Can you work these out from the model? Positions are in its coordinate system, mm. Give positions to 0.01 mm unless a question says otherwise; leave off trailing zeros. Loops run counter-clockwise (first coordinate to the right, second up) from the corner with the lowest first, then second, coordinate; pieces in that order, holes last. Notation, with made-up numbers: (56, -16.5) - (61, -16.5) arc R13 cw to (61, -8.5) - close; hole circle Ø8 at (15.5, 61.25). An arc over 180 degrees is marked (long way). Answer as a JSON object with one key per item and string values.
```python
from build123d import *

# Parameters (mm, degrees)
F0_R     = 6.35
F1_DEPTH = 2.54
F2_DEPTH = 25.4


with BuildPart() as f1:
    # F0 (on Top) → F1 (new body)
    with BuildSketch(Plane.XY):
        with BuildLine():
            ThreePointArc((1.98040625, 18.6275212343), (3.3011106094, 18.4393390607), (4.6050729167, 18.157639155))
            ThreePointArc((4.6050729167, 18.157639155), (6.310350892, 21.0006716461), (8.2563229167, 23.6846983968))
            ThreePointArc((8.2563229167, 23.6846983968), (6.9543084231, 24.0991576742), (5.63165625, 24.4421000352))
            ThreePointArc((5.63165625, 24.4421000352), (3.6830183734, 21.6120562584), (1.98040625, 18.6275212343))
        make_face()
        with BuildLine():
            ThreePointArc((8.2563229167, -23.6846983968), (6.310350892, -21.0006716461), (4.6050729167, -18.157639155))
            ThreePointArc((4.6050729167, -18.157639155), (3.3011106094, -18.4393390607), (1.98040625, -18.6275212343))
            ThreePointArc((1.98040625, -18.6275212343), (3.6830183734, -21.6120562584), (5.63165625, -24.4421000352))
            ThreePointArc((5.63165625, -24.4421000352), (6.9543084231, -24.0991576742), (8.2563229167, -23.6846983968))
        make_face()
        with BuildLine():
            ThreePointArc((1.98040625, -18.6275212343), (-18.7325, 0), (1.98040625, 18.6275212343))
            ThreePointArc((1.98040625, 18.6275212343), (3.6830183734, 21.6120562584), (5.63165625, 24.4421000352))
            ThreePointArc((5.63165625, 24.4421000352), (-25.0825, 0), (5.63165625, -24.4421000352))
            ThreePointArc((5.63165625, -24.4421000352), (3.6830183734, -21.6120562584), (1.98040625, -18.6275212343))
        make_face()
        with BuildLine():
            ThreePointArc((5.63165625, 24.4421000352), (6.9543084231, 24.0991576742), (8.2563229167, 23.6846983968))
            ThreePointArc((8.2563229167, 23.6846983968), (50.64125, 35.9767570584), (76.2, 0))
            ThreePointArc((76.2, 0), (50.64125, -35.9767570584), (8.2563229167, -23.6846983968))
            ThreePointArc((8.2563229167, -23.6846983968), (6.9543084231, -24.0991576742), (5.63165625, -24.4421000352))
            ThreePointArc((5.63165625, -24.4421000352), (50.9859634875, -38.5429830838), (78.74, 0))
            ThreePointArc((78.74, 0), (50.9859634875, 38.5429830838), (5.63165625, 24.4421000352))
        make_face()
        with BuildLine():
            ThreePointArc((-1.8626666667, 7.388834339), (-0.3539283859, 13.1493342679), (1.98040625, 18.6275212343))
            ThreePointArc((1.98040625, 18.6275212343), (-18.7325, 0), (1.98040625, -18.6275212343))
            ThreePointArc((1.98040625, -18.6275212343), (-0.3539283859, -13.1493342679), (-1.8626666667, -7.388834339))
            ThreePointArc((-1.8626666667, -7.388834339), (-7.62, 0), (-1.8626666667, 7.388834339))
        make_face()
        with BuildLine():
            ThreePointArc((0.762, 7.5818042708), (2.2909514135, 13.012380233), (4.6050729167, 18.157639155))
            ThreePointArc((4.6050729167, 18.157639155), (3.3011106094, 18.4393390607), (1.98040625, 18.6275212343))
            ThreePointArc((1.98040625, 18.6275212343), (-0.3539283859, 13.1493342679), (-1.8626666667, 7.388834339))
            ThreePointArc((-1.8626666667, 7.388834339), (-0.5587272379, 7.5994883955), (0.762, 7.5818042708))
        make_face()
        with BuildLine():
            ThreePointArc((4.6050729167, -18.157639155), (14.7846387284, -11.5030871473), (18.7325, 0))
            ThreePointArc((18.7325, 0), (14.7846387284, 11.5030871473), (4.6050729167, 18.157639155))
            ThreePointArc((4.6050729167, 18.157639155), (2.2909514135, 13.012380233), (0.762, 7.5818042708))
            ThreePointArc((0.762, 7.5818042708), (5.6511432472, 5.1116513966), (7.62, 0))
            ThreePointArc((7.62, 0), (5.6511432472, -5.1116513966), (0.762, -7.5818042708))
            ThreePointArc((0.762, -7.5818042708), (2.2909514135, -13.012380233), (4.6050729167, -18.157639155))
        make_face()
        with BuildLine():
            ThreePointArc((1.98040625, -18.6275212343), (3.3011106094, -18.4393390607), (4.6050729167, -18.157639155))
            ThreePointArc((4.6050729167, -18.157639155), (2.2909514135, -13.012380233), (0.762, -7.5818042708))
            ThreePointArc((0.762, -7.5818042708), (-0.5587272379, -7.5994883955), (-1.8626666667, -7.388834339))
            ThreePointArc((-1.8626666667, -7.388834339), (-0.3539283859, -13.1493342679), (1.98040625, -18.6275212343))
        make_face()
        with BuildLine():
            ThreePointArc((4.6050729167, 18.157639155), (14.7846387284, 11.5030871473), (18.7325, 0))
            ThreePointArc((18.7325, 0), (14.7846387284, -11.5030871473), (4.6050729167, -18.157639155))
            ThreePointArc((4.6050729167, -18.157639155), (6.310350892, -21.0006716461), (8.2563229167, -23.6846983968))
            ThreePointArc((8.2563229167, -23.6846983968), (20.4477508031, -14.5265719751), (25.0825, 0))
            ThreePointArc((25.0825, 0), (20.4477508031, 14.5265719751), (8.2563229167, 23.6846983968))
            ThreePointArc((8.2563229167, 23.6846983968), (6.310350892, 21.0006716461), (4.6050729167, 18.157639155))
        make_face()
        with BuildLine():
            ThreePointArc((76.2, 0), (50.64125, 35.9767570584), (8.2563229167, 23.6846983968))
            ThreePointArc((8.2563229167, 23.6846983968), (20.4477508031, 14.5265719751), (25.0825, 0))
            ThreePointArc((25.0825, 0), (20.4477508031, -14.5265719751), (8.2563229167, -23.6846983968))
            ThreePointArc((8.2563229167, -23.6846983968), (50.64125, -35.9767570584), (76.2, 0))
        make_face()
        with Locations((38.1, 0)):
            Circle(F0_R, mode=Mode.SUBTRACT)
        with Locations((38.1, 0)):
            Circle(F0_R)
    extrude(amount=F1_DEPTH)

    # F0 (on Top) → F2 (join)
    with BuildSketch(Plane.XY):
        with BuildLine():
            ThreePointArc((5.63165625, 24.4421000352), (6.9543084231, 24.0991576742), (8.2563229167, 23.6846983968))
            ThreePointArc((8.2563229167, 23.6846983968), (50.64125, 35.9767570584), (76.2, 0))
            ThreePointArc((76.2, 0), (50.64125, -35.9767570584), (8.2563229167, -23.6846983968))
            ThreePointArc((8.2563229167, -23.6846983968), (6.9543084231, -24.0991576742), (5.63165625, -24.4421000352))
            ThreePointArc((5.63165625, -24.4421000352), (50.9859634875, -38.5429830838), (78.74, 0))
            ThreePointArc((78.74, 0), (50.9859634875, 38.5429830838), (5.63165625, 24.4421000352))
        make_face()
        with BuildLine():
            ThreePointArc((1.98040625, 18.6275212343), (3.3011106094, 18.4393390607), (4.6050729167, 18.157639155))
            ThreePointArc((4.6050729167, 18.157639155), (6.310350892, 21.0006716461), (8.2563229167, 23.6846983968))
            ThreePointArc((8.2563229167, 23.6846983968), (6.9543084231, 24.0991576742), (5.63165625, 24.4421000352))
            ThreePointArc((5.63165625, 24.4421000352), (3.6830183734, 21.6120562584), (1.98040625, 18.6275212343))
        make_face()
        with BuildLine():
            ThreePointArc((1.98040625, -18.6275212343), (-18.7325, 0), (1.98040625, 18.6275212343))
            ThreePointArc((1.98040625, 18.6275212343), (3.6830183734, 21.6120562584), (5.63165625, 24.4421000352))
            ThreePointArc((5.63165625, 24.4421000352), (-25.0825, 0), (5.63165625, -24.4421000352))
            ThreePointArc((5.63165625, -24.4421000352), (3.6830183734, -21.6120562584), (1.98040625, -18.6275212343))
        make_face()
        with BuildLine():
            ThreePointArc((8.2563229167, -23.6846983968), (6.310350892, -21.0006716461), (4.6050729167, -18.157639155))
            ThreePointArc((4.6050729167, -18.157639155), (3.3011106094, -18.4393390607), (1.98040625, -18.6275212343))
            ThreePointArc((1.98040625, -18.6275212343), (3.6830183734, -21.6120562584), (5.63165625, -24.4421000352))
            ThreePointArc((5.63165625, -24.4421000352), (6.9543084231, -24.0991576742), (8.2563229167, -23.6846983968))
        make_face()
    extrude(amount=F2_DEPTH)


solid = f1.part
```
1) I need wall thicknesses on L1, parallel to Y at x = 0, z = 14.75; L2, parallel to X at y = -0.5, z = 17.75; L3, parallel to Z at x = 35, y = 19.5. Which ranges of each line are inside material? Lowest first, please.
Check sheet entries:
{"L1": "-25.08 to -18.73, 18.73 to 25.08", "L2": "-25.08 to -18.73, 76.2 to 78.74", "L3": "0 to 2.54"}
2) If we mould it in two halves opening along Y, with no side actions, what happens to faces 1 (the flat face through (39, 1, 2.54)), 2 (the flat face through (26, 1, 0)), 3 (the cylindrical face through (78.715, -1.42, 12.522))? For each: released by +Y, released by -Y, zero draft, split by the parting line, or undercut.
Check sheet entries:
{"face 1": "undercut", "face 2": "zero draft", "face 3": "split by the parting line"}
3) Imagine slicing it at D-D on y = -21.5. Write out the boundary of the cut face in (x, z).
Check sheet entries:
{"outline": "(-12.92, 0) - (72.59, 0) - (72.59, 25.4) - (69.55, 25.4) - (69.55, 2.54) - (6.65, 2.54) - (6.65, 25.4) - (-12.92, 25.4) - close"}
4) Imagine slicing it at A-A on x = 38.1. Write out the boundary of the cut face in (y, z), and give its area (3 significant figures).
Check sheet entries:
{"outline": "(-40.64, 0) - (40.64, 0) - (40.64, 25.4) - (38.1, 25.4) - (38.1, 2.54) - (-38.1, 2.54) - (-38.1, 25.4) - (-40.64, 25.4) - close", "area": "323 mm2"}
5) Imagine slicing it at B-B on y = -4. Write out the boundary of the cut face in (x, z), and give its area (3 significant figures).
Check sheet entries:
{"outline": "(-24.76, 0) - (-6.49, 0) - (-6.49, 2.54) - (-18.3, 2.54) - (-18.3, 25.4) - (-24.76, 25.4) - close; (6.49, 0) - (78.54, 0) - (78.54, 25.4) - (75.99, 25.4) - (75.99, 2.54) - (6.49, 2.54) - close", "area": "436 mm2"}
6) I'm going to push flat-ended pins straight in: P1, Ø8, axis at x = 6, z = 4, coming from the +Y side; P2, Ø6, axis at x = 18.5, z = 3.5, coming from the -Y side; P3, Ø1, axis at y = -20.5, z = 11, coming from the +X side. Where does each tip first touch, or does it pass through?
Check sheet entries:
{"P1": "y = 29.36", "P2": "y = -37.1", "P3": "x = 73.48"}
7) Imagine slicing it at C-C on z = 20.25. Write out the boundary of the cut face in (x, y) (1 decimal), and give its area (3 significant figures).
Check sheet entries:
{"outline": "(5.6, -24.4) arc R40.6 ccw (long way) to (5.6, 24.4) arc R25.1 ccw (long way) to start; hole (4.6, -18.2) arc R38.1 ccw (long way) to (4.6, 18.2) arc R18.7 ccw (long way) to start", "area": "1,020 mm2"}
